Autodesk Inventor part; units mm, degrees
ref_plane "YZ Plane" through (0, 0, 0) normal (1, 0, 0) x (0, 1, 0)
ref_plane "XZ Plane" through (0, 0, 0) normal (0, 1, 0) x (-1, 0, 0)
ref_plane "XY Plane" through (0, 0, 0) normal (0, 0, 1) x (1, 0, 0)
sketch "Sketch1" plane through (0, 0, 0) normal (0, 1, 0) x (-1, 0, 0)
  circle A0 centre (0, 0) radius 20.75
  dimension "d0" = 41.5
extrude "Extrusion1" add sketch "Sketch1" along normal blind 1.5
sketch "Sketch2" plane through (0, 1.5, 0) normal (0, 1, 0) x (1, 0, 0)
  circle A0 centre (0, 0) radius 19
  dimension "d3" = 38
extrude "Extrusion2" add sketch "Sketch2" along normal blind 8
sketch "Sketch3" plane through (0, 9.5, 0) normal (0, 1, 0) x (1, 0, 0)
  circle A0 centre (0, 0) radius 20.75
extrude "Extrusion3" add sketch "Sketch3" along normal blind 1.5
sketch "Sketch4" plane through (0, 11, 0) normal (0, 1, 0) x (1, 0, 0)
  line L0 (0, 0) -> (-15, 0)
  circle A0 centre (-15, 0) radius 1.6
  line L1 (0, 0) -> (15, 0)
  circle A1 centre (15, 0) radius 1.6
  dimension "d8" = 15
  dimension "d9" = 3.2
  dimension "d10" = 15
hole "Hole1" at (-15, 11, 0) at (15, 11, 0) direction (0, -1, 0) diameter 3 depth 8 tip angle 118 counterbore diameter 3.2 counterbore depth 6
sketch "Sketch5" plane through (0, 0, 0) normal (0, -1, 0) x (1, 0, 0)
  line L0 (0, 0) -> (-4.8, 0)
  circle A0 centre (-4.8, 0) radius 11
  dimension "d18" = 4.8
  dimension "d19" = 22
extrude "Extrusion4" add sketch "Sketch5" along normal blind 5
sketch "Sketch6" plane through (-4.8, -5, 0) normal (0, -1, 0) x (1, 0, 0)
  circle A0 centre (0, 0) radius 6
  point P0 (4.8, 0)
  dimension "d22" = 12
extrude "Extrusion5" cut sketch "Sketch6" against normal through all
sketch "Sketch8" plane through (0, 0, 0) normal (1, 0, 0) x (0, 1, 0)
  line L0 (-5, -6) -> (-5, 6)
  line L1 (-5, 0) -> (-2.5, 0)
  circle A0 centre (-2.5, 0) radius 1.5
  point P0 (0, 0)
  dimension "d25" = 2.5
  dimension "d26" = 3
extrude "Extrusion6" cut sketch "Sketch8" against normal through all
sketch "Sketch9" plane through (0, 0, 0) normal (0, 0, 1) x (1, 0, 0)
  line L0 (6.2, 0) -> (6.2, -5)
  line L1 (6.2, -2.5) -> (-4.8, -2.5)
  circle A0 centre (-4.8, -2.5) radius 1.5
  point P0 (0, 0)
  dimension "d29" = 11
  dimension "d30" = 3
extrude "Extrusion7" cut sketch "Sketch9" against normal through all
properties part number "Assieme eccentrico"
Could you check a few things on this model? Use its own coordinates, in mm. A direction names the side the tool comes from. Give positions to 0.01 mm unless a question says otherwise; leave off trailing zeros. Loops run counter-clockwise (first coordinate to the right, second up) from the corner with the lowest first, then second, coordinate; pieces in that order, holes last. Notation, with made-up numbers: M -15.5,7.5 L 21.5,7.5 A16 ccw 21.5,37.5 Z; hole C 36.25,-12 d10. An arc over 180 degrees is marked long. Answer as a JSON object with one key per item and string values.
Q1. If I drill on probe 1 along X at (y, z) = (3.9, 0), over which ranges is the centre line in solid material (lowest first)? Write a range as [from, to].
Values found:
{"probe 1": "x = [-19, -16.5], [-13.5, -10.8], [1.2, 13.5], [16.5, 19]"}
Q2. For P1, Ø1.8, axis at x = 15, z = 0, coming from the +Y side; P2, Ø3.5, axis at y = -2.5, z = 0, coming from the +X side; P3, Ø1, axis at x = 15, z = 0.5, coming from the +Y side; P4, Ø1, axis at x = -2, z = 3, coming from the -Y side, each with a flat end and sliding along its axis, tell me the tip position at first contact or that it passes through.
Values found:
{"P1": "stops at y = 2.64", "P2": "stops at x = 6.2", "P3": "stops at y = 2.7", "P4": "passes through"}
Q3. If we mould it in two halves opening along Z, with no side actions, what happens to faces 4 (the flat face through (9, 9.5, 17)), 5 (the cylindrical face through (-19.8, 0.7, -6.2)), 6 (the conical face through (15.258, 2.255, -0.034))? For each: pulls with the +Z half, pulls with the -Z half, needs draft (parallel to the pull), parting line crosses it, or undercut.
Values found:
{"face 4": "needs draft", "face 5": "parting line crosses it", "face 6": "undercut"}
Q4. Suppose I cut it at B-B, the plane y = -2.5. List the corners of the cut face in (x, z) for me.
Values found:
{"outline": "M -15.7,-1.5 A11 ccw -6.3,-10.9 L -6.3,-5.81 A6 cw -10.61,-1.5 Z; M -15.7,1.5 L -10.61,1.5 A6 cw long -3.3,-5.81 L -3.3,-10.9 A11 ccw long Z"}
Q5. Suppose I cut it at D-D, the plane x = -4.8. List the corners of the cut face in (y, z) for me.
Values found:
{"outline": "M -5,-11 L -4,-11 L -4,-6 L -5,-6 Z; M -5,6 L 11,6 L 11,20.19 L 9.5,20.19 L 9.5,18.38 L 1.5,18.38 L 1.5,20.19 L 0,20.19 L 0,11 L -5,11 Z; M -1,-11 L 0,-11 L 0,-20.19 L 1.5,-20.19 L 1.5,-18.38 L 9.5,-18.38 L 9.5,-20.19 L 11,-20.19 L 11,-6 L -1,-6 Z"}
Q6. Suppose I cut it at C-C, the plane z = -7. List the corners of the cut face in (x, y) for me, plus the area to 3 significant figures.
Values found:
{"outline": "M -19.53,0 L -13.29,0 L -13.29,-5 L 3.69,-5 L 3.69,0 L 19.53,0 L 19.53,1.5 L 17.66,1.5 L 17.66,9.5 L 19.53,9.5 L 19.53,11 L -19.53,11 L -19.53,9.5 L -17.66,9.5 L -17.66,1.5 L -19.53,1.5 Z; hole C -4.8,-2.5 d3", "area": "478 mm²"}
Q7. Suppose I cut it at A-A, the plane x = -0.5. List the corners of the cut face in (y, z) for me, plus the area to 3 significant figures.
Values found:
{"outline": "M -5,-10.12 L 0,-10.12 L 0,-20.74 L 1.5,-20.74 L 1.5,-18.99 L 9.5,-18.99 L 9.5,-20.74 L 11,-20.74 L 11,-4.18 L -5,-4.18 Z; M -5,4.18 L 11,4.18 L 11,20.74 L 9.5,20.74 L 9.5,18.99 L 1.5,18.99 L 1.5,20.74 L 0,20.74 L 0,10.12 L -5,10.12 Z", "area": "396 mm²"}
Q8. For faces 1 (the cylindrical face through (13.414, 7.958, -0.208)), 2 (the cylindrical face through (-4.995, -1.013, -8.368)), 3 (the cylindrical face through (8.767, 5.444, -16.856)), which set-ups out of +Z, -Z, +X, -X, +Y, -Y let a thin tool reach every point of the face, with its end or its side?
Values found:
{"face 1": "+Y", "face 2": "-Z", "face 3": "none"}
